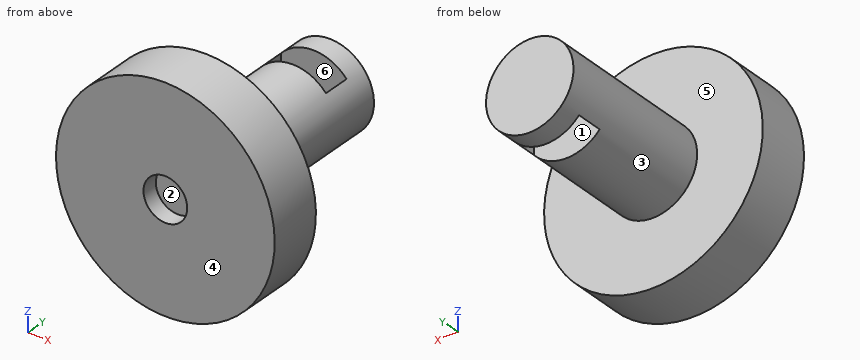
from build123d import *

# Parameters (mm, degrees)
SKETCH2_R               = 20
BOSS_EXTRUDE1_DEPTH     = 10
SKETCH3_R               = 8
BOSS_EXTRUDE2_DEPTH     = 30
CUT_EXTRUDE1_DEPTH      = 49.989794856
CUT_EXTRUDE1_DEPTH_BACK = 49.989794856
SKETCH4_W               = 12
SKETCH4_H               = 5
SKETCH5_R               = 4
CUT_EXTRUDE2_DEPTH      = 3


with BuildPart() as part:
    # Sketch2 → Boss-Extrude1 (new body)
    with BuildSketch(Plane(origin=(0, 0, 0), x_dir=(1, 0, 0), z_dir=(0, 1, 0))):
        with Locations(Location((0, 0, 0), (0, 0, 270))):
            Circle(SKETCH2_R)
    extrude(amount=BOSS_EXTRUDE1_DEPTH)

    # Sketch3 → Boss-Extrude2 (add)
    with BuildSketch(Plane(origin=(0, 10, 0), x_dir=(1, 0, 0), z_dir=(0, 1, 0))):
        with Locations(Location((0, 0, 0), (0, 0, 270))):
            Circle(SKETCH3_R)
    extrude(amount=BOSS_EXTRUDE2_DEPTH)

    # Sketch4 → Cut-Extrude1 (cut, two sides: drawn at the far end of the back side and taken through both)
    with BuildSketch(Plane.XY.offset(-CUT_EXTRUDE1_DEPTH_BACK)):
        with Locations((0, 33.5)):
            Rectangle(SKETCH4_W, SKETCH4_H)
    extrude(amount=CUT_EXTRUDE1_DEPTH + CUT_EXTRUDE1_DEPTH_BACK, mode=Mode.SUBTRACT)

    # Sketch5 → Cut-Extrude2 (cut)
    with BuildSketch(Plane.XZ):
        with Locations(Location((0, 0, 0), (0, 0, 270))):
            Circle(SKETCH5_R)
    extrude(amount=-CUT_EXTRUDE2_DEPTH, mode=Mode.SUBTRACT)


solid = part.part
Here's how the part is built. I have some questions about the finished solid (model axes, mm). Face numbers are marked on the shaded views. A direction names the side the tool comes from. Coordinates: 2 decimals unless noted, no trailing zeros. Loops run counter-clockwise (first coordinate to the right, second up) from the corner with the lowest first, then second, coordinate; pieces in that order, holes last.
1. Imagine slicing it at D-D, the plane y = 33.5. Please give me the cut outline in (x, z), and give its area (3 significant figures).
2. Imagine slicing it at B-B, the plane z = 6. Please give me the cut outline in (x, y).
3. If we mould it in two halves opening along Z, with no side actions, what happens to the marked faces 1, 2 and 3? For each: pulls with the +Z half, pulls with the -Z half, needs draft (parallel to the pull), parting line crosses it, or undercut.
4. For the marked faces 4, 5 and 6, which set-ups out of +Z, -Z, +X, -X, +Y, -Y let a thin tool reach every point of the face, with its end or its side?
5. I need wall thicknesses on L1, parallel to X at y = 1, z = 0; L2, parallel to Y at x = 8.5, z = -15.5; L3, parallel to X at y = 13, z = 6. Which ranges of each line are inside material? Lowest first, please.
6. Imagine slicing it at A-A, the plane x = 0. Please give me the cut outline in (y, z).
7. Imagine slicing it at C-C, the plane z = 0. Please give me the cut outline in (x, y), and give its area (3 significant figures).
8. For P1, Ø1.5, axis at y = 34, z = 1.5, coming from the -X side; P2, Ø4, axis at x = -12.5, z = -11, coming from the -Y side; P3, Ø2.5, axis at x = -1.5, z = 1.5, coming from the -Y side; P4, Ø3, axis at y = 26.5, z = 3.5, coming from the +X side, each with a flat end and sliding along its axis, tell me the tip position at first contact or that it passes through.
Taken from the geometry:
1. outline: (-6, -5.29) - (-6, 5.29) arc R8 ccw to start; (6, -5.29) arc R8 ccw to (6, 5.29) - close
1. area: 29.0 mm2
2. outline: (-19.08, 0) - (19.08, 0) - (19.08, 10) - (5.29, 10) - (5.29, 31) - (-5.29, 31) - (-5.29, 10) - (-19.08, 10) - close; (-5.29, 36) - (5.29, 36) - (5.29, 40) - (-5.29, 40) - close
3. face 1: needs draft
3. face 2: undercut
3. face 3: parting line crosses it
4. face 4: +Z, -Z, +X, -X, -Y
4. face 5: +Y
4. face 6: +Z, -Z
5. L1: x = -20 to -4, 4 to 20
5. L2: y = 0 to 10
5. L3: x = -5.29 to 5.29
6. outline: (0, -20) - (10, -20) - (10, -8) - (31, -8) - (31, 8) - (10, 8) - (10, 20) - (0, 20) - (0, 4) - (3, 4) - (3, -4) - (0, -4) - close; (36, -8) - (40, -8) - (40, 8) - (36, 8) - close
7. outline: (-20, 0) - (-4, 0) - (-4, 3) - (4, 3) - (4, 0) - (20, 0) - (20, 10) - (8, 10) - (8, 40) - (-8, 40) - (-8, 10) - (-20, 10) - close; hole (-6, 31) - (6, 31) - (6, 36) - (-6, 36) - close
7. area: 796 mm2
8. P1: stops at x = -7.96
8. P2: stops at y = 0
8. P3: stops at y = 3
8. P4: stops at x = 7.75
